```python
from build123d import *

# Parameters (mm, degrees)
SKETCH1_W           = 755.65
SKETCH1_H           = 88.9
BOSS_EXTRUDE1_DEPTH = 38.1
SKETCH2_W           = 88.9
SKETCH2_H           = 38.1
CUT_EXTRUDE1_DEPTH  = 39.1


with BuildPart() as part:
    # Sketch1 → Boss-Extrude1 (new body)
    with BuildSketch(Plane(origin=(0, 0, 0), x_dir=(1, 0, 0), z_dir=(0, 1, 0))):
        with Locations((377.825, 44.45)):
            Rectangle(SKETCH1_W, SKETCH1_H)
    extrude(amount=BOSS_EXTRUDE1_DEPTH)

    # Sketch2 → Cut-Extrude1 (cut, through all)
    with BuildSketch(Plane.XZ):
        with Locations((711.2, -69.85)):
            Rectangle(SKETCH2_W, SKETCH2_H)
    extrude(amount=-CUT_EXTRUDE1_DEPTH, mode=Mode.SUBTRACT)


solid = part.part
```
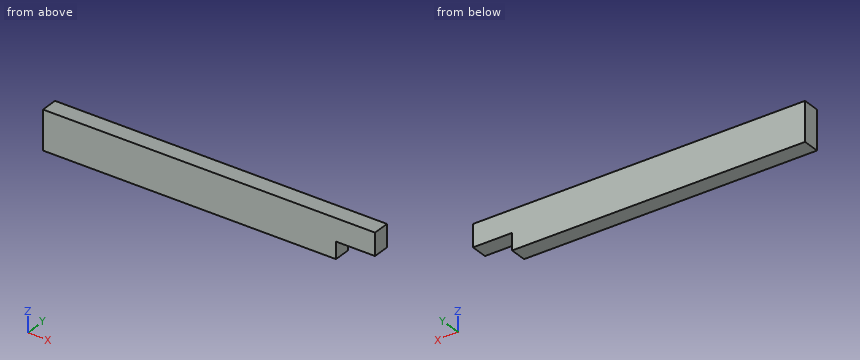
CAD build for the part. Positions are in the model's coordinates, mm. Round coordinates to 2 decimals unless told otherwise and drop trailing zeros. Loops run counter-clockwise (first coordinate to the right, second up) from the corner with the lowest first, then second, coordinate; pieces in that order, holes last. Notation, with made-up numbers: M 89.5,-19.5 L 111.5,-19.5 A21 cw 111.5,-11.5 Z; hole C -8,8.5 d10. An arc over 180 degrees is marked long. Use a Markdown table: item, result. Add a question column.
(1) Cut at B-B (x = 675.5). Give the cut face in (y, z).
(2) Cut at A-A (y = 13). Give the cut face in (x, z).
(3) Cut at C-C (z = -77.5). Give the cut face in (x, y).
(4) Drill centre lines: line 1 (Z direction, x = 717.5, y = 6); line 2 (X direction, y = 20, z = -73.5). Where is each one in solid material? Low to high.
(5) Flat gauge pins, fed straight in: pin 1 (11.5 mm diameter, centred on y = 10.5, z = -62, fed in from +X); pin 2 (19 mm diameter, centred on x = 715, y = 18, fed in from -Z). Where does each tip first touch, or does it go through?
Geometry says:
| question | item | result |
|---|---|---|
| 1 | outline | M 0,-50.8 L 38.1,-50.8 L 38.1,0 L 0,0 Z |
| 2 | outline | M 0,-88.9 L 666.75,-88.9 L 666.75,-50.8 L 755.65,-50.8 L 755.65,0 L 0,0 Z |
| 3 | outline | M 0,0 L 666.75,0 L 666.75,38.1 L 0,38.1 Z |
| 4 | line 1 | z = -50.8 to 0 |
| 4 | line 2 | x = 0 to 666.75 |
| 5 | pin 1 | stops at x = 666.75 |
| 5 | pin 2 | stops at z = -50.8 |
